```python
from build123d import *

# Parameters (mm, degrees)
SKETCH1_W                  = 524
SKETCH1_H                  = 180
BOSS_EXTRUDE1_DEPTH        = 3
SKETCH2_W                  = 444
SKETCH2_H                  = 10
TRACKS_DEPTH               = 4
SKETCH3_R                  = 2.5
SCREW_MOUNTING_HOLES_DEPTH = 4


with BuildPart() as part:
    # Sketch1 → Boss-Extrude1 (new body)
    with BuildSketch(Plane(origin=(0, 0, 0), x_dir=(1, 0, 0), z_dir=(0, 1, 0))):
        with Locations((262, 90)):
            Rectangle(SKETCH1_W, SKETCH1_H)
    extrude(amount=BOSS_EXTRUDE1_DEPTH)

    # Sketch2 → Tracks (cut, through all)
    with BuildSketch(Plane.XZ):
        with BuildLine():
            ThreePointArc((484, -65), (489, -70), (484, -75))
            Line((484, -75), (484, -65))
        make_face()
        with Locations((262, -70)):
            Rectangle(SKETCH2_W, SKETCH2_H)
        with BuildLine():
            ThreePointArc((40, -75), (35, -70), (40, -65))
            Line((40, -65), (40, -75))
        make_face()
    tracks = extrude(amount=-TRACKS_DEPTH, mode=Mode.SUBTRACT)

    # Sketch3 → screw mounting holes (cut, through all)
    with BuildSketch(Plane.XZ):
        with Locations((6, -80)):
            Circle(SKETCH3_R)
        with Locations((518, -80)):
            Circle(SKETCH3_R)
    screw_mounting_holes = extrude(amount=-SCREW_MOUNTING_HOLES_DEPTH, mode=Mode.SUBTRACT)

    # Mirror2: Tracks, screw mounting holes across plane
    add(tracks.mirror(Plane(origin=(0, 0, -90), x_dir=(1, 0, 0), z_dir=(0, 0, -1))), mode=Mode.SUBTRACT)
    add(screw_mounting_holes.mirror(Plane(origin=(0, 0, -90), x_dir=(1, 0, 0), z_dir=(0, 0, -1))), mode=Mode.SUBTRACT)


solid = part.part
```
Read the model definition and answer for the solid it produces. Units are mm, in the model's axes. Coordinates: 2 decimals unless noted, no trailing zeros. Write each loop counter-clockwise with the first axis right and the second up, starting at its lowest first coordinate (ties: lowest second). Pieces come first, ordered by that corner, then holes. Notation, with made-up numbers: (8.25, -6.75) -> (58.25, -6.75) arc R11 cw to (58.25, 9.25) -> close; hole circle Ø7 at (-25, 21.25). An arc over 180 degrees is marked (long way). Write item = value, one per line.
(1) Section B-B on y = 0.85 is taken. Write down the section's boundary in (x, z).
From the geometry:
outline = (0, -180) -> (524, -180) -> (524, 0) -> (0, 0) -> close; hole circle Ø5 at (6, -100); hole circle Ø5 at (6, -80); hole (40, -115) -> (484, -115) arc R5 ccw to (484, -105) -> (40, -105) arc R5 ccw to start; hole (40, -75) -> (484, -75) arc R5 ccw to (484, -65) -> (40, -65) arc R5 ccw to start; hole circle Ø5 at (518, -100); hole circle Ø5 at (518, -80)
(2) Section C-C on z = -70 is taken. Write down the section's boundary in (x, y), plus the area to 3 significant figures.
From the geometry:
outline = (0, 0) -> (35, 0) -> (35, 3) -> (0, 3) -> close; (489, 0) -> (524, 0) -> (524, 3) -> (489, 3) -> close
area = 210 mm2
(3) Section A-A on x = 425.5 is taken. Write down the section's boundary in (y, z).
From the geometry:
outline = (0, -180) -> (3, -180) -> (3, -115) -> (0, -115) -> close; (0, -105) -> (3, -105) -> (3, -75) -> (0, -75) -> close; (0, -65) -> (3, -65) -> (3, 0) -> (0, 0) -> close
(4) Straight lines are drawn through the part: L1, parallel to Z at x = 138.5, y = 0.95; L2, parallel to Z at x = 518, y = 1.65; L3, parallel to X at y = 2.05, z = -100. For each, find the intervals that lie inside material, in ascending order. Write a range as from..to.
From the geometry:
L1 = -180..-115, -105..-75, -65..0
L2 = -180..-102.5, -97.5..-82.5, -77.5..0
L3 = 0..3.5, 8.5..515.5, 520.5..524
